Design review of the part shown in the three views and the two pictorial views. Dimensions are in mm from the part's minimum x, y and z. Coordinates: 2 decimals unless noted, no trailing zeros. Loops run counter-clockwise (first coordinate to the right, second up) from the corner with the lowest first, then second, coordinate; pieces in that order, holes last. Notation, with made-up numbers: (-37, -34) - (-1, -34) arc R26 cw to (-1, -3) - close; hole circle Ø2 at (2, -40). An arc over 180 degrees is marked (long way). One line per question, with ' | ' between items.
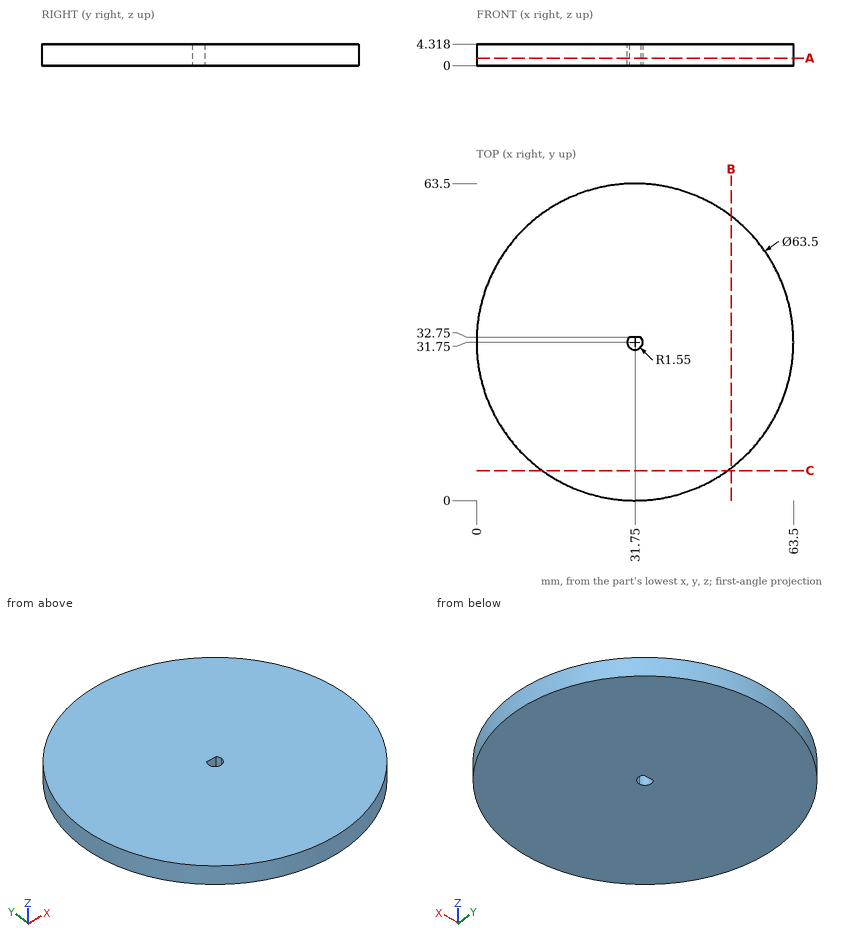
Q1. Take a section at A-A (z = 1.5). Give the boundary of the cut face in (x, y), plus the area to 3 significant figures.
Returned:
outline: circle Ø63.5 at (31.75, 31.75); hole (30.57, 32.75) arc R1.55 ccw to (31.75, 30.2) arc R1.55 ccw to (33.3, 31.75) arc R1.55 ccw to (32.93, 32.75) - close | area: 3,160 mm²
Q2. To check wall thickness, follow line 1 along Y through (x, z) = (31.5, 3.45); line 2 along Y through (x, z) = (19.5, 0.25); line 3 along X through (y, z) = (16, 0.35). State the ranges of each line that lie inside material, in increasing order.
Returned:
line 1: y = 0 to 30.22, 32.75 to 63.5 | line 2: y = 2.46 to 61.04 | line 3: x = 4.18 to 59.32
Q3. For pin 1 (1.5 mm diameter, centred on y = 17.5, z = 3, fed in from +X); pin 2 (1.5 mm diameter, centred on y = 18.5, z = 1, fed in from +X); pin 3 (1.5 mm diameter, centred on x = 38.5, z = 0.5, fed in from -Y), all flat-tipped, find the tip position at first contact; note any pin that passes through.
Returned:
pin 1: stops at x = 60.49 | pin 2: stops at x = 60.94 | pin 3: stops at y = 0.57
Q4. Take a section at B-B (x = 51). Give the boundary of the cut face in (y, z), plus the area to 3 significant figures.
Returned:
outline: (6.5, 0) - (57, 0) - (57, 4.32) - (6.5, 4.32) - close | area: 218 mm²
Q5. Take a section at C-C (y = 6). Give the boundary of the cut face in (x, z).
Returned:
outline: (13.18, 0) - (50.32, 0) - (50.32, 4.32) - (13.18, 4.32) - close
